CAD build for the part. Positions are in the model's coordinates, mm. A direction names the side the tool comes from. Give positions to 0.01 mm unless a question says otherwise; leave off trailing zeros. Order: outer loops, then holes, each group sorted by start corner. A loop starts at its lowest first (then second) coordinate and runs counter-clockwise, first axis right, second up. Notation, with made-up numbers: (55.25, 25.25) -> (60.25, 25.25) arc R21 ccw to (60.25, 60.25) -> close; hole circle Ø6 at (89, -29). An arc over 180 degrees is marked (long way). Use one line per item in the form item = value. Start each with the question number.
1) Drop flat-ended pins along their axis: P1, Ø15, axis at x = -2, y = -7, coming from the +Z side; P2, Ø3, axis at y = -19, z = 2.5, coming from the +X side; P3, Ø1.3, axis at x = 9.5, z = -1, coming from the +Y side. Give the stop position or say it passes through.
2) Probe line 1 (Z direction, x = 0, y = -34.5); line 2 (X direction, y = -34, z = -2); line 3 (X direction, y = -26.5, z = 8). List the from-to ranges inside material, lowest first.
3) Cut at B-B, the plane x = 0. Give the cut face in (y, z), and give its area (3 significant figures).
4) Mould opens along Z. For faces 5 (the face through (-15.47, -10.11, -7.86)), 6 (the face through (0, -10, 13)), 7 (the face through (0, -20, 0)) say: pulls with the +Z half, pulls with the -Z half, needs draft (parallel to the pull), parting line crosses it, or undercut.
5) Cut at A-A, the plane y = -10. Give the cut face in (x, z), and give its area (3 significant figures).
6) Cut at C-C, the plane y = -33. Give the cut face in (x, z), and give its area (3 significant figures).
7) Tool access for faces 1 (the face through (-8, -40, -2)), 2 (the face through (21.24, -10.11, 1.7)), 3 (the face through (-15.19, -21.01, 7.43)), 4 (the face through (15.33, -10.11, -8)): list every direction of +Z, -Z, +X, -X, +Y, -Y with a clear straight run to the whole face (end or side of a thin tool).
8) Cut at D-D, the plane z = 9.5. Give the cut face in (x, y), and give its area (3 significant figures).
from build123d import *

# Parameters (mm, degrees)
F0_W      = 39
F0_H      = 22
F1_DEPTH  = 20
F2_SIZE   = 10
F3_R      = 1.5
F5_DEPTH  = 20
F6_T      = -2
F7_R      = 2.25
F8_DEPTH  = 1.5
F10_R     = 2.25
F11_DEPTH = 20
F13_DEPTH = 1
F14_R     = 30
F15_DEPTH = 5
F16_R     = 22
F17_DEPTH = 20
F18_R     = 2.25
F19_DEPTH = 20


with BuildPart() as f1:
    # F0 (on Front) → F1 (new body)
    with BuildSketch(Plane.XZ):
        Rectangle(F0_W, F0_H)
    extrude(amount=F1_DEPTH)

    # F2
    f2_edges = [f1.edges().sort_by_distance(p)[0] for p in [
        (19.5, -10, 11),
        (-19.5, -10, 11),
        (19.5, -10, -11),
        (-19.5, -10, -11),
    ]]
    chamfer(f2_edges, length=F2_SIZE)

    # F3
    f3_edges = [f1.edges().sort_by_distance(p)[0] for p in [
        (19.5, -10, -1),
        (-19.5, -10, 1),
        (-19.5, -10, -1),
        (19.5, -10, 1),
    ]]
    fillet(f3_edges, radius=F3_R)

    # F4 (on face) → F5 (join, through all)
    with BuildSketch(Plane.XZ.offset(20)):
        with BuildLine():
            ThreePointArc((-20.4748737342, 2.8535533906), (-21.2335783638, 1.7180716697), (-21.5, 0.3786796564))
            Line((-21.5, 0.3786796564), (-21.5, -0.3786796564))
            ThreePointArc((-21.5, -0.3786796564), (-21.2335783638, -1.7180716697), (-20.4748737342, -2.8535533906))
            Line((-20.4748737342, -2.8535533906), (-10.3284271247, -13))
            Line((-10.3284271247, -13), (10.3284271247, -13))
            Line((10.3284271247, -13), (20.4748737342, -2.8535533906))
            ThreePointArc((20.4748737342, -2.8535533906), (21.2335783638, -1.7180716697), (21.5, -0.3786796564))
            Line((21.5, -0.3786796564), (21.5, 0.3786796564))
            ThreePointArc((21.5, 0.3786796564), (21.2335783638, 1.7180716697), (20.4748737342, 2.8535533906))
            Line((20.4748737342, 2.8535533906), (10.3284271247, 13))
            Line((10.3284271247, 13), (-10.3284271247, 13))
            Line((-10.3284271247, 13), (-20.4748737342, 2.8535533906))
        make_face()
    extrude(amount=-F5_DEPTH)

    # F6
    f6_openings = [f1.faces().sort_by_distance(p)[0] for p in [
        (0, -20, 0),
        (0, 0, 0),
    ]]
    offset(amount=F6_T, openings=f6_openings)

    # F7 (on face) → F8 (join)
    with BuildSketch(Plane.XZ.offset(20)):
        with BuildLine():
            Line((10.3284271247, 13), (-10.3284271247, 13))
            Line((-10.3284271247, 13), (-20.4748737342, 2.8535533906))
            ThreePointArc((-20.4748737342, 2.8535533906), (-21.2335783638, 1.7180716697), (-21.5, 0.3786796564))
            Line((-21.5, 0.3786796564), (-21.5, -0.3786796564))
            ThreePointArc((-21.5, -0.3786796564), (-21.2335783638, -1.7180716697), (-20.4748737342, -2.8535533906))
            Line((-20.4748737342, -2.8535533906), (-10.3284271247, -13))
            Line((-10.3284271247, -13), (10.3284271247, -13))
            Line((10.3284271247, -13), (20.4748737342, -2.8535533906))
            ThreePointArc((20.4748737342, -2.8535533906), (21.2335783638, -1.7180716697), (21.5, -0.3786796564))
            Line((21.5, -0.3786796564), (21.5, 0.3786796564))
            ThreePointArc((21.5, 0.3786796564), (21.2335783638, 1.7180716697), (20.4748737342, 2.8535533906))
            Line((20.4748737342, 2.8535533906), (10.3284271247, 13))
        make_face()
        with Locations((-8.5, -2)):
            Circle(F7_R, mode=Mode.SUBTRACT)
        with Locations((8.5, -2)):
            Circle(F7_R, mode=Mode.SUBTRACT)
        with Locations((0, 3)):
            Circle(F7_R, mode=Mode.SUBTRACT)
    extrude(amount=F8_DEPTH)

    # F10 (on face) → F11 (join)
    with BuildSketch(Plane.XZ.offset(21.5)):
        with BuildLine():
            ThreePointArc((-21.5, -0.3786796564), (-21.2335783638, -1.7180716697), (-20.4748737342, -2.8535533906))
            Line((-20.4748737342, -2.8535533906), (-10.3284271247, -13))
            Line((-10.3284271247, -13), (10.3284271247, -13))
            Line((10.3284271247, -13), (20.4748737342, -2.8535533906))
            ThreePointArc((20.4748737342, -2.8535533906), (21.2335783638, -1.7180716697), (21.5, -0.3786796564))
            Line((21.5, -0.3786796564), (21.5, 0.3786796564))
            ThreePointArc((21.5, 0.3786796564), (21.2335783638, 1.7180716697), (20.4748737342, 2.8535533906))
            Line((20.4748737342, 2.8535533906), (10.3284271247, 13))
            Line((10.3284271247, 13), (-10.3284271247, 13))
            Line((-10.3284271247, 13), (-20.4748737342, 2.8535533906))
            ThreePointArc((-20.4748737342, 2.8535533906), (-21.2335783638, 1.7180716697), (-21.5, 0.3786796564))
            Line((-21.5, 0.3786796564), (-21.5, -0.3786796564))
        make_face()
        with Locations((-8.5, -2)):
            Circle(F10_R, mode=Mode.SUBTRACT)
        with Locations((8.5, -2)):
            Circle(F10_R, mode=Mode.SUBTRACT)
        with Locations((0, 3)):
            Circle(F10_R, mode=Mode.SUBTRACT)
    extrude(amount=F11_DEPTH)

    # F12 (on offset) → F13 (cut)
    with BuildSketch(Plane.XZ.offset(21.5)):
        with BuildLine():
            Line((20.4748737342, 2.8535533906), (10.3284271247, 13))
            Line((10.3284271247, 13), (-10.3284271247, 13))
            Line((-10.3284271247, 13), (-20.4748737342, 2.8535533906))
            ThreePointArc((-20.4748737342, 2.8535533906), (-21.2335783638, 1.7180716697), (-21.5, 0.3786796564))
            Line((-21.5, 0.3786796564), (-21.5, -0.3786796564))
            ThreePointArc((-21.5, -0.3786796564), (-21.2335783638, -1.7180716697), (-20.4748737342, -2.8535533906))
            Line((-20.4748737342, -2.8535533906), (-10.3284271247, -13))
            Line((-10.3284271247, -13), (10.3284271247, -13))
            Line((10.3284271247, -13), (20.4748737342, -2.8535533906))
            ThreePointArc((20.4748737342, -2.8535533906), (21.2335783638, -1.7180716697), (21.5, -0.3786796564))
            Line((21.5, -0.3786796564), (21.5, 0.3786796564))
            ThreePointArc((21.5, 0.3786796564), (21.2335783638, 1.7180716697), (20.4748737342, 2.8535533906))
        make_face()
        with BuildLine():
            Line((-10.1213203436, 12.5), (10.1213203436, 12.5))
            Line((10.1213203436, 12.5), (20.1213203436, 2.5))
            ThreePointArc((20.1213203436, 2.5), (20.7716385975, 1.5267299535), (21, 0.3786796564))
            Line((21, 0.3786796564), (21, -0.3786796564))
            ThreePointArc((21, -0.3786796564), (20.7716385975, -1.5267299535), (20.1213203436, -2.5))
            Line((20.1213203436, -2.5), (10.1213203436, -12.5))
            Line((10.1213203436, -12.5), (-10.1213203436, -12.5))
            Line((-10.1213203436, -12.5), (-20.1213203436, -2.5))
            ThreePointArc((-20.1213203436, -2.5), (-20.7716385975, -1.5267299535), (-21, -0.3786796564))
            Line((-21, -0.3786796564), (-21, 0.3786796564))
            ThreePointArc((-21, 0.3786796564), (-20.7716385975, 1.5267299535), (-20.1213203436, 2.5))
            Line((-20.1213203436, 2.5), (-10.1213203436, 12.5))
        make_face(mode=Mode.SUBTRACT)
    extrude(amount=-F13_DEPTH, mode=Mode.SUBTRACT)

    # F14 (on face) → F15 (join)
    with BuildSketch(Plane.XZ.offset(41.5)):
        Circle(F14_R)
    extrude(amount=F15_DEPTH)

    # F16 (on face) → F17 (join, through all)
    with BuildSketch(Plane(origin=(0, -41.5, 0), x_dir=(-1, 0, 0), z_dir=(0, 1, 0))):
        Circle(F16_R)
    extrude(amount=F17_DEPTH)

    # F18 (on face) → F19 (cut)
    with BuildSketch(Plane(origin=(0, -20, 0), x_dir=(-1, 0, 0), z_dir=(0, 1, 0))):
        with Locations((8.5, -2)):
            Circle(F18_R)
        with Locations((0, 3)):
            Circle(F18_R)
        with Locations((-8.5, -2)):
            Circle(F18_R)
    extrude(amount=-F19_DEPTH, mode=Mode.SUBTRACT)


solid = f1.part
Result:
q1.P1 = 13
q1.P2 = 21.44
q1.P3 = -40
q2.line_1 = -22 to 0.75, 5.25 to 22
q2.line_2 = -21.91 to -10.75, -6.25 to 6.25, 10.75 to 21.91
q2.line_3 = -20.49 to 20.49
q3.outline = (-46.5, -30) -> (-41.5, -30) -> (-41.5, -22) -> (-21.5, -22) -> (-21.5, -12.5) -> (-20.5, -12.5) -> (-20.5, -13) -> (0, -13) -> (0, -11) -> (-20, -11) -> (-20, 0.75) -> (-40, 0.75) -> (-40, 5.25) -> (-20, 5.25) -> (-20, 11) -> (0, 11) -> (0, 13) -> (-20.5, 13) -> (-20.5, 12.5) -> (-21.5, 12.5) -> (-21.5, 22) -> (-41.5, 22) -> (-41.5, 30) -> (-46.5, 30) -> close
q3.area = 1,210 mm²
q4.face_5 = pulls with the -Z half
q4.face_6 = pulls with the +Z half
q4.face_7 = undercut
q5.outline = (-21.5, -0.38) arc R3.5 ccw to (-20.47, -2.85) -> (-10.33, -13) -> (10.33, -13) -> (20.47, -2.85) arc R3.5 ccw to (21.5, -0.38) -> (21.5, 0.38) arc R3.5 ccw to (20.47, 2.85) -> (10.33, 13) -> (-10.33, 13) -> (-20.47, 2.85) arc R3.5 ccw to (-21.5, 0.38) -> close; hole (-19.5, -0.38) arc R1.5 ccw to (-19.06, -1.44) -> (-9.5, -11) -> (9.5, -11) -> (19.06, -1.44) arc R1.5 ccw to (19.5, -0.38) -> (19.5, 0.38) arc R1.5 ccw to (19.06, 1.44) -> (9.5, 11) -> (-9.5, 11) -> (-19.06, 1.44) arc R1.5 ccw to (-19.5, 0.38) -> close
q5.area = 210 mm²
q6.outline = circle Ø44 at (0, 0); hole circle Ø4.5 at (-8.5, -2); hole circle Ø4.5 at (0, 3); hole circle Ø4.5 at (8.5, -2)
q6.area = 1,470 mm²
q7.face_1 = +Y
q7.face_2 = +Z, +X, +Y
q7.face_3 = +Z, -X
q7.face_4 = -Z, +X, +Y
q8.outline = (-28.46, -46.5) -> (28.46, -46.5) -> (28.46, -41.5) -> (19.84, -41.5) -> (19.84, -21.5) -> (13.12, -21.5) -> (13.12, -20.5) -> (13.83, -20.5) -> (13.83, 0) -> (11, 0) -> (11, -20) -> (-11, -20) -> (-11, 0) -> (-13.83, 0) -> (-13.83, -20.5) -> (-13.12, -20.5) -> (-13.12, -21.5) -> (-19.84, -21.5) -> (-19.84, -41.5) -> (-28.46, -41.5) -> close
q8.area = 1,230 mm²
